Design review of the part built by this model. Coordinates are the model's own, in mm. Face numbers are marked on the shaded views. A direction names the side the tool comes from. Give positions to 0.01 mm unless a question says otherwise; leave off trailing zeros. Loops run counter-clockwise (first coordinate to the right, second up) from the corner with the lowest first, then second, coordinate; pieces in that order, holes last. Notation, with made-up numbers: (56, 2.5) - (70, 2.5) arc R24 ccw to (70, 31.5) - close; hole circle Ø2 at (14, 39.5). An arc over 180 degrees is marked (long way). One line per item, written item: value. Start each with the question number.
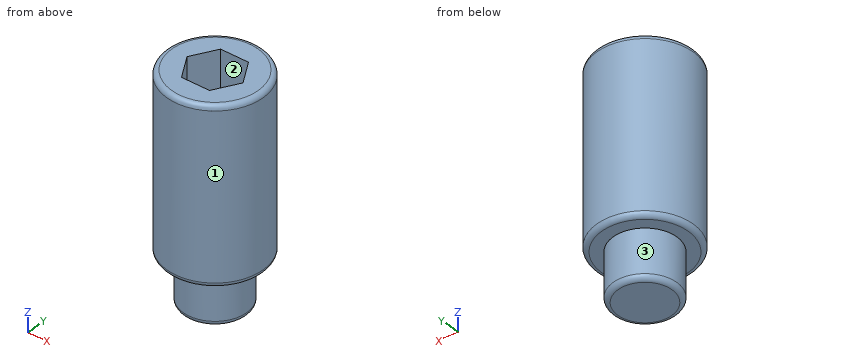
Autodesk Inventor part; units mm, degrees
ref_plane "YZ Plane" through (0, 0, 0) normal (1, 0, 0) x (0, 1, 0)
ref_plane "XZ Plane" through (0, 0, 0) normal (0, 1, 0) x (-1, 0, 0)
ref_plane "XY Plane" through (0, 0, 0) normal (0, 0, 1) x (1, 0, 0)
sketch "Esquisse1" plane through (0, 0, 0) normal (0, 0, 1) x (1, 0, 0)
  circle A0 centre (0, 0) radius 2.5
  dimension "d0" = 5
extrude "Extrusion1" add sketch "Esquisse1" along normal blind 9
sketch "Esquisse2" plane through (0, 0, 0) normal (0, 0, -1) x (-1, 0, 0)
  circle A0 centre (0, 0) radius 2.5
  circle A1 centre (0, 0) radius 1.65
  dimension "d3" = 3.3
extrude "Extrusion2" add sketch "Esquisse2" along normal blind 2.5 contours A1
thread "Filetage1"
sketch "Esquisse3" plane through (0, 0, 9) normal (0, 0, 1) x (1, 0, 0)
  line L0 (0.7217, 1.25) -> (1.4434, 0)
  line L1 (1.4434, 0) -> (0.7217, -1.25)
  line L2 (0.7217, -1.25) -> (-0.7217, -1.25)
  line L3 (-0.7217, -1.25) -> (-1.4434, 0)
  line L4 (-1.4434, 0) -> (-0.7217, 1.25)
  line L5 (-0.7217, 1.25) -> (0.7217, 1.25)
  point P0 (0, 0)
  point P1 (0, 0)
  dimension "d8" = 2.5
extrude "Extrusion3" cut sketch "Esquisse3" against normal blind 2.5
fillet "Congé1" radius 0.25 3 edges at (-2.5, 0, 9) (-2.5, 0, 0) (1.65, 0, -2.5)
properties part number "M5 pour ressort" material "----------"
(1) To check wall thickness, follow L1, parallel to Z at x = 1.65, y = -0.4; L2, parallel to Z at x = -0.2, y = -0.6; L3, parallel to X at y = 1, z = 7.25. State the ranges of each line that lie inside material, in increasing order. Write a range as from..to.
(2) Take a section at A-A on x = 0. State the section outline as (y, z) points, and give its area (3 significant figures).
(3) For pin 1 Ø1.3 at (x, y) = (0, -0.5) entering from +Z; pin 2 Ø1 at (y, z) = (-0.5, 3.5) entering from -X, all flat-tipped, find the tip position at first contact; note any pin that passes through.
(4) Machinability: for the marked faces 1, 2 and 3, which of the approach directions +Z, -Z, +X, -X, +Y, -Y give a long, thin tool a straight path to every point of the face, cutting with its end or side? Answer none if there is none.
(5) Take a section at C-C on z = 2. State the section outline as (x, y) points.
(6) Take a section at B-B on z = -0.5. State the section outline as (x, y) points.
Here are the results:
1. L1: 0..9
1. L2: -2.5..6.5
1. L3: -2.29..-0.87, 0.87..2.29
2. outline: (-2.5, 0.25) arc R0.25 ccw to (-2.25, 0) - (-1.65, 0) - (-1.65, -2.25) arc R0.25 ccw to (-1.4, -2.5) - (1.4, -2.5) arc R0.25 ccw to (1.65, -2.25) - (1.65, 0) - (2.25, 0) arc R0.25 ccw to (2.5, 0.25) - (2.5, 8.75) arc R0.25 ccw to (2.25, 9) - (1.25, 9) - (1.25, 6.5) - (-1.25, 6.5) - (-1.25, 9) - (-2.25, 9) arc R0.25 ccw to (-2.5, 8.75) - close
2. area: 46.9 mm²
3. pin 1: z = 6.5
3. pin 2: x = -2.5
4. face 1: +Z, -Z
4. face 2: +Z
4. face 3: -Z
5. outline: circle Ø5 at (0, 0)
6. outline: circle Ø3.3 at (0, 0)
